Part print with two shaded views. Sizes in mm from the minimum x, y, z corner. Round coordinates to 2 decimals unless told otherwise and drop trailing zeros. Order: outer loops, then holes, each group sorted by start corner. A loop starts at its lowest first (then second) coordinate and runs counter-clockwise, first axis right, second up. Notation, with made-up numbers: (73, -36.75) - (96, -36.75) arc R9 ccw to (96, -29.75) - close; hole circle Ø5 at (67.5, 83). An arc over 180 degrees is marked (long way). Write item = value, one per line.
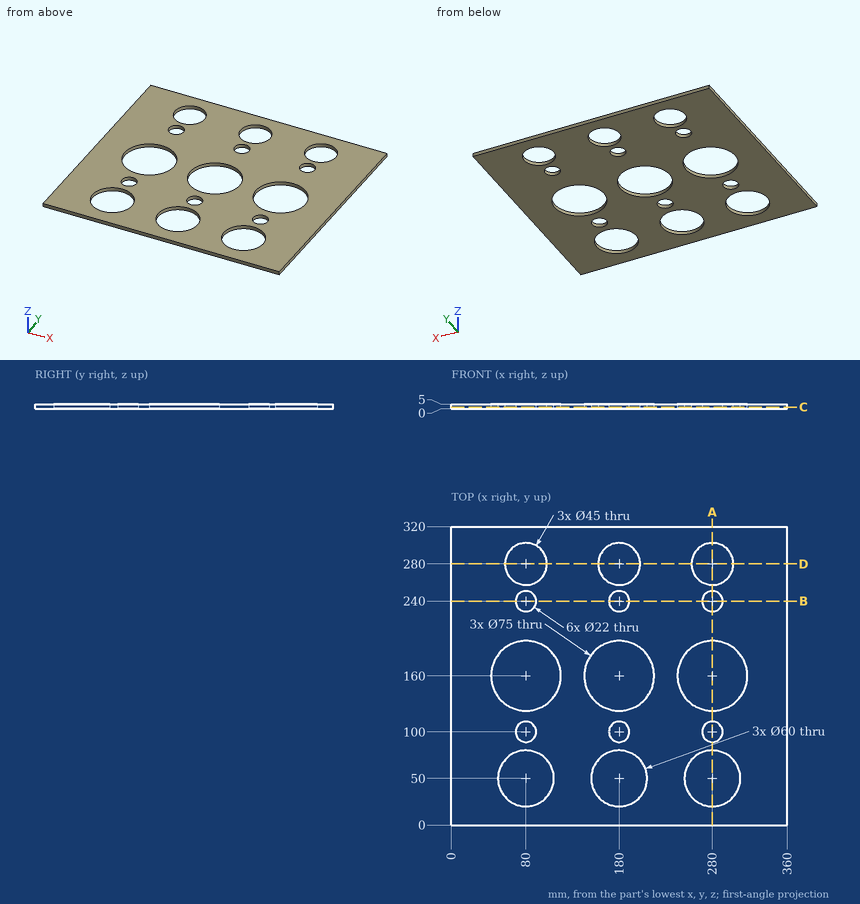
1) Cut at B-B (y = 240). Write the cut outline in (x, z).
Conclusion:
outline = (0, 0) - (69, 0) - (69, 5) - (0, 5) - close; (91, 0) - (169, 0) - (169, 5) - (91, 5) - close; (191, 0) - (269, 0) - (269, 5) - (191, 5) - close; (291, 0) - (360, 0) - (360, 5) - (291, 5) - close
2) Flat gauge pins, fed straight in: pin 1 Ø20 at (x, y) = (180, 240) entering from -Z; pin 2 Ø1 at (x, y) = (318, 212) entering from -Z. Where does each tip first touch, or does it go through?
Conclusion:
pin_1 = through
pin_2 = 0
3) Cut at C-C (z = 1.65). Give the number of separate pieces and of enclosed holes in the cut face, and give its area (3 significant figures).
Conclusion:
separate_pieces = 1
enclosed_holes = 15
area = 86,400 mm^2
4) Wall check: line 1 along Y through (x, z) = (280, 2.75); line 2 along X through (y, z) = (259.5, 1.9); line 3 along Y through (x, z) = (264.5, 1.8). Give the ranges that are in metal, low to high.
Conclusion:
line_1 = 0 to 20, 80 to 89, 111 to 122.5, 197.5 to 229, 251 to 257.5, 302.5 to 320
line_2 = 0 to 70.73, 89.27 to 170.73, 189.27 to 270.73, 289.27 to 360
line_3 = 0 to 24.31, 75.69 to 125.85, 194.15 to 263.69, 296.31 to 320
5) Cut at D-D (y = 280). Write the cut outline in (x, z).
Conclusion:
outline = (0, 0) - (57.5, 0) - (57.5, 5) - (0, 5) - close; (102.5, 0) - (157.5, 0) - (157.5, 5) - (102.5, 5) - close; (202.5, 0) - (257.5, 0) - (257.5, 5) - (202.5, 5) - close; (302.5, 0) - (360, 0) - (360, 5) - (302.5, 5) - close
6) Cut at A-A (x = 280). Write the cut outline in (y, z).
Conclusion:
outline = (0, 0) - (20, 0) - (20, 5) - (0, 5) - close; (80, 0) - (89, 0) - (89, 5) - (80, 5) - close; (111, 0) - (122.5, 0) - (122.5, 5) - (111, 5) - close; (197.5, 0) - (229, 0) - (229, 5) - (197.5, 5) - close; (251, 0) - (257.5, 0) - (257.5, 5) - (251, 5) - close; (302.5, 0) - (320, 0) - (320, 5) - (302.5, 5) - close
